Input: dimensioned drawing with shaded views. Units: mm. Origin: part minimum x, y, z. Round coordinates to 2 decimals unless told otherwise and drop trailing zeros. Loops run counter-clockwise (first coordinate to the right, second up) from the corner with the lowest first, then second, coordinate; pieces in that order, holes last.
1) Section A-A, the plane z = 0.85. Return loops of the section in (x, y), and give its area (3 significant figures).
2) First-contact query: pin 1 (1.6 mm diameter, centred on y = 9, z = 1, fed in from -X); pin 2 (1.5 mm diameter, centred on x = 22, z = 0.5, fed in from -Y). Flat tips, straight axial feed; report the tip coordinate or a pass-through.
3) Ray query, line 1 along X through (y, z) = (30.5, 0.6); line 2 along Y through (x, z) = (4.5, 2.7); line 3 along Y through (x, z) = (12.5, 1.7) (1 decimal). Return the intervals inside material, ascending.
4) Section B-B, the plane y = 39. Return loops of the section in (x, z).
5) Section C-C, the plane x = 2. Return loops of the section in (y, z).
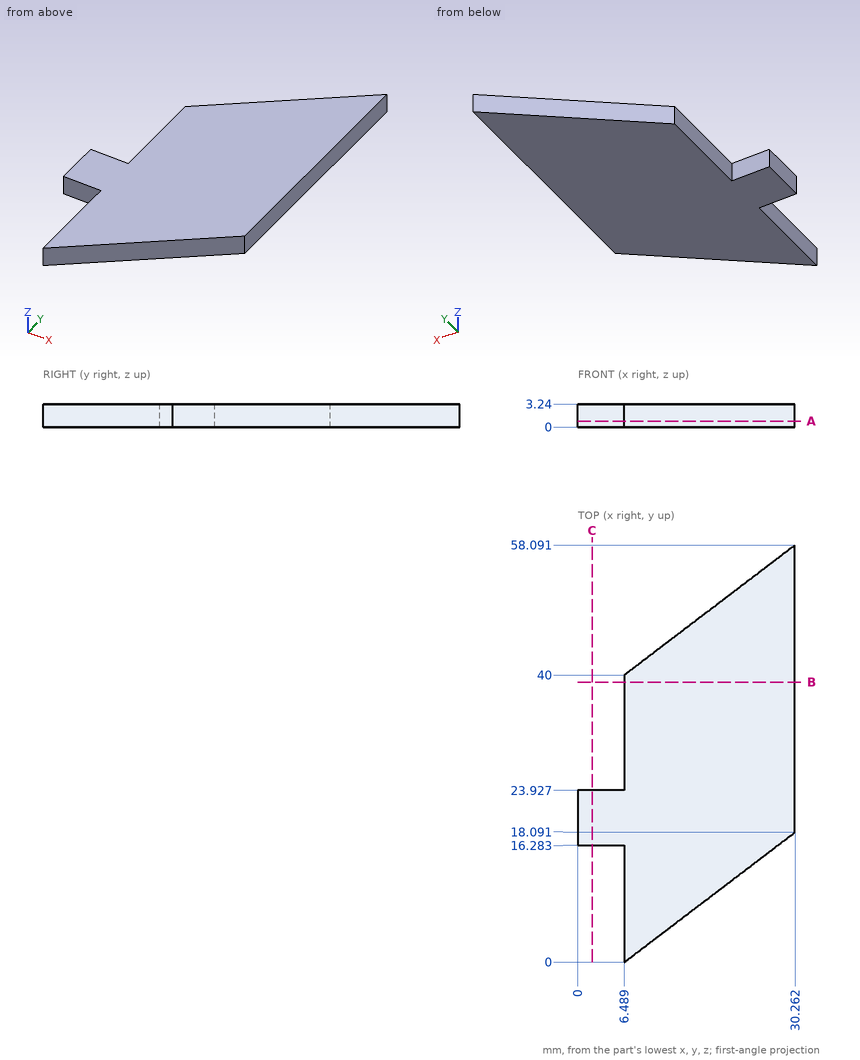
Final values:
1. outline: (0, 16.28) - (6.49, 16.28) - (6.49, 0) - (30.26, 18.09) - (30.26, 58.09) - (6.49, 40) - (6.49, 23.93) - (0, 23.93) - close
1. area: 1,000 mm2
2. pin 1: stops at x = 6.49
2. pin 2: stops at y = 11.23
3. line 1: x = 6.49 to 30.26
3. line 2: y = 16.28 to 23.93
3. line 3: y = 4.6 to 44.6
4. outline: (6.49, 0) - (30.26, 0) - (30.26, 3.24) - (6.49, 3.24) - close
5. outline: (16.28, 0) - (23.93, 0) - (23.93, 3.24) - (16.28, 3.24) - close
